Build history of the part. All positions in model axes, mm. Face numbers are marked on the shaded views. A direction names the side the tool comes from. Coordinates: 2 decimals unless noted, no trailing zeros. Loops run counter-clockwise (first coordinate to the right, second up) from the corner with the lowest first, then second, coordinate; pieces in that order, holes last.
(1) Wall check: L1, parallel to Z at x = 9, y = 0; L2, parallel to X at y = 2.5, z = -1.75; L3, parallel to Y at x = -7.5, z = -0.25. Give the ranges that are in metal, low to high.
(2) Slice it at A-A (y = 0). Give the cut face in (x, z).
(3) Slice it at C-C (x = 14.5). Give the cut face in (y, z).
(4) Tool access for the marked faces 1, 2 and 3: list every direction of +Z, -Z, +X, -X, +Y, -Y with a clear straight run to the whole face (end or side of a thin tool).
(5) Flat gauge pins, fed straight in: P1, Ø5, axis at x = -8.5, z = -1.5, coming from the -Y side; P2, Ø1, axis at x = -3, y = 1.5, coming from the +Z side; P3, Ø5, axis at x = 3, y = -3, coming from the -Z side; P4, Ø2, axis at x = -11, z = -3.5, coming from the +Y side. Where does each tip first touch, or does it go through?
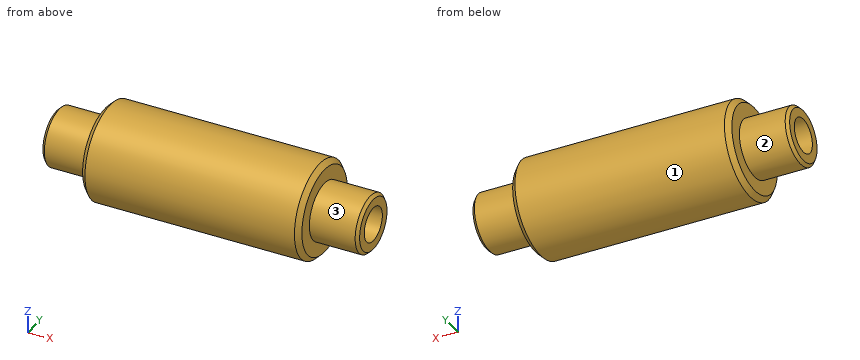
Autodesk Inventor part; units mm, degrees
ref_plane "YZ Plane" through (0, 0, 0) normal (1, 0, 0) x (0, 1, 0)
ref_plane "XZ Plane" through (0, 0, 0) normal (0, 1, 0) x (-1, 0, 0)
ref_plane "XY Plane" through (0, 0, 0) normal (0, 0, 1) x (1, 0, 0)
sketch "Эскиз2" plane through (0, 0, 0) normal (0, 0, 1) x (1, 0, 0)
  line L0 (0, 4.9) -> (11.25, 4.9)
  line L1 (11.25, 4.9) -> (11.25, 2.95)
  line L2 (11.25, 2.95) -> (16.25, 2.95)
  line L3 (16.25, 2.95) -> (16.25, 1.75)
  line L4 (16.25, 1.75) -> (0, 1.75)
  line L5 (0, 0) -> (17.7021, 0) construction
  line L6 (0, 0) -> (0, 8.5432) construction
  line L7 (0, 4.9) -> (-11.25, 4.9)
  line L8 (-11.25, 4.9) -> (-11.25, 2.95)
  line L9 (-11.25, 2.95) -> (-16.25, 2.95)
  line L10 (-16.25, 2.95) -> (-16.25, 1.75)
  line L11 (-16.25, 1.75) -> (0, 1.75)
  dimension "d3" = 9.8
  dimension "d4" = 22.5
  dimension "d6" = 5.9
  dimension "d7" = 3.5
  dimension "d12" = 5
revolve "Вращение1" add sketch "Эскиз2" angle 360 about axis through (0, 0, 0) along (1, 0, 0)
chamfer "Фаска1" distance 0.5 angle 45 2 edges at (-11.25, -4.9, 0) (11.25, -4.9, 0)
chamfer "Фаска2" distance 0.3 angle 45 2 edges at (-16.25, -2.95, 0) (16.25, -2.95, 0)
properties part number "Ось двусторонняя"
Response values:
1. L1: z = -4.9 to -1.75, 1.75 to 4.9
1. L2: x = -11.25 to 11.25
1. L3: y = -4.89 to -1.73, 1.73 to 4.89
2. outline: (-16.25, -2.65) - (-15.95, -2.95) - (-11.25, -2.95) - (-11.25, -4.4) - (-10.75, -4.9) - (10.75, -4.9) - (11.25, -4.4) - (11.25, -2.95) - (15.95, -2.95) - (16.25, -2.65) - (16.25, -1.75) - (-16.25, -1.75) - close; (-16.25, 1.75) - (16.25, 1.75) - (16.25, 2.65) - (15.95, 2.95) - (11.25, 2.95) - (11.25, 4.4) - (10.75, 4.9) - (-10.75, 4.9) - (-11.25, 4.4) - (-11.25, 2.95) - (-15.95, 2.95) - (-16.25, 2.65) - close
3. outline: circle Ø5.9 at (0, 0); hole circle Ø3.5 at (0, 0)
4. face 1: +X, -X
4. face 2: -X
4. face 3: +X
5. P1: stops at y = -4.9
5. P2: stops at z = 4.8
5. P3: stops at z = -4.87
5. P4: stops at y = 4.2
